Input: part model. Units: mm. Frame: model coordinates. A direction names the side the tool comes from. Give positions to 0.01 mm unless a question says otherwise; leave off trailing zeros. Write each loop counter-clockwise with the first axis right and the second up, starting at its lowest first coordinate (ties: lowest second). Pieces come first, ordered by that corner, then holes.
```python
from build123d import *

# Parameters (mm, degrees)
SKETCH1_W           = 58.42
SKETCH1_H           = 33.02
BOSS_EXTRUDE1_DEPTH = 7.62
BOSS_EXTRUDE2_DEPTH = 3.81
CUT_EXTRUDE1_DEPTH  = 35.407391648


with BuildPart() as part:
    # Sketch1 → Boss-Extrude1 (new body)
    with BuildSketch(Plane(origin=(0, 0, 0), x_dir=(1, 0, 0), z_dir=(0, 1, 0))):
        Rectangle(SKETCH1_W, SKETCH1_H)
    extrude(amount=BOSS_EXTRUDE1_DEPTH)

    # Sketch2 → Boss-Extrude2 (add)
    with BuildSketch(Plane.XZ):
        Polygon((5.08, -2.932939367), (5.08, 2.932939367), (0, 5.865878735), (-5.08, 2.932939367), (-5.08, -2.932939367), (0, -5.865878735), align=None)
    extrude(amount=BOSS_EXTRUDE2_DEPTH)

    # Sketch3 → Cut-Extrude1 (cut, through all)
    with BuildSketch(Plane(origin=(0, 0, 0), x_dir=(-1, 0, 0), z_dir=(0, -1, 0))):
        Polygon((26.162, -13.462), (26.162, 13.462), (8.128, 0), align=None)
        Polygon((8.128, -13.462), (21.066651169, -13.462), (8.128, -3.803570254), align=None)
        Polygon((21.066651169, 13.462), (8.128, 3.803570254), (8.128, 13.462), align=None)
        Polygon((-21.066651169, -13.462), (-8.128, -3.803570254), (-8.128, -13.462), align=None)
        Polygon((-8.128, 13.462), (-21.066651169, 13.462), (-8.128, 3.803570254), align=None)
        Polygon((-8.128, 0), (-26.162, -13.462), (-26.162, 13.462), align=None)
    extrude(amount=-CUT_EXTRUDE1_DEPTH, mode=Mode.SUBTRACT)


solid = part.part
```
Item 1: Section C-C (z = -11.5). Return loops of the section in (x, y).
Item 2: Pin query (flat end, axial travel): pin 1 (1.1 mm diameter, centred on y = -3, z = 0, fed in from +X); pin 2 (1.9 mm diameter, centred on y = -1, z = 0, fed in from -X). Return the tip coordinate at first contact, or that it passes through.
Item 3: Section B-B (x = -12.5). Return loops of the section in (y, z).
Item 4: Set-up query: faces 4 (the flat face through (-5.08, -2, 0)), 5 (the flat face through (2.576, -1.878, 4.379)), 6 (the flat face through (8.128, 4, -9)). Return all of +Z, -Z, +X, -X, +Y, -Y with unobstructed straight access to the full face (end or side cutting, diameter ignored); none if empty.
Item 5: Ray query, line 1 (Z direction, x = 16.5, y = 1.25); line 2 (Z direction, x = -14, y = 5); line 3 (X direction, y = 0.25, z = 3). Return the intervals inside material, ascending.
Item 6: Mould query, pull axis Z, two halves, no side actions, for faces 1 (the flat face through (14.69, 3.76, 8.7)), 2 (the flat face through (-7, 0, 0)), 3 (the flat face through (-2.576, -1.878, -4.379)). Classes: +Z half, -Z half, draft (parallel to the pull), parting line (faces both ways), or undercut.
Item 7: Section A-A (y = 6). Return loops of the section in (x, z), and give its area (3 significant figures).
Item 8: Section D-D (y = -2.5). Return loops of the section in (x, z).
Solved:
1. outline: (-29.21, 0) - (-26.16, 0) - (-26.16, 7.62) - (-29.21, 7.62) - close; (-23.53, 0) - (-18.44, 0) - (-18.44, 7.62) - (-23.53, 7.62) - close; (-8.13, 0) - (8.13, 0) - (8.13, 7.62) - (-8.13, 7.62) - close; (18.44, 0) - (23.53, 0) - (23.53, 7.62) - (18.44, 7.62) - close; (26.16, 0) - (29.21, 0) - (29.21, 7.62) - (26.16, 7.62) - close
2. pin 1: stops at x = 5.08
2. pin 2: stops at x = -5.08
3. outline: (0, -16.51) - (7.62, -16.51) - (7.62, -13.46) - (0, -13.46) - close; (0, -7.07) - (7.62, -7.07) - (7.62, -3.26) - (0, -3.26) - close; (0, 3.26) - (7.62, 3.26) - (7.62, 7.07) - (0, 7.07) - close; (0, 13.46) - (7.62, 13.46) - (7.62, 16.51) - (0, 16.51) - close
4. face 4: +Z, -Z, -X, -Y
4. face 5: +Z, +X, -Y
4. face 6: +Y, -Y
5. line 1: z = -16.51 to -13.46, -10.05 to -6.25, 6.25 to 10.05, 13.46 to 16.51
5. line 2: z = -16.51 to -13.46, -8.19 to -4.38, 4.38 to 8.19, 13.46 to 16.51
5. line 3: x = -29.21 to -26.16, -12.15 to 12.15, 26.16 to 29.21
6. face 1: undercut
6. face 2: draft
6. face 3: -Z half
7. outline: (-29.21, -16.51) - (29.21, -16.51) - (29.21, 16.51) - (-29.21, 16.51) - close; hole (-26.16, -13.46) - (-8.13, 0) - (-26.16, 13.46) - close; hole (-21.07, -13.46) - (-8.13, -13.46) - (-8.13, -3.8) - close; hole (-21.07, 13.46) - (-8.13, 3.8) - (-8.13, 13.46) - close; hole (8.13, -13.46) - (21.07, -13.46) - (8.13, -3.8) - close; hole (8.13, 0) - (26.16, -13.46) - (26.16, 13.46) - close; hole (8.13, 3.8) - (21.07, 13.46) - (8.13, 13.46) - close
7. area: 1,190 mm2
8. outline: (-5.08, -2.93) - (0, -5.87) - (5.08, -2.93) - (5.08, 2.93) - (0, 5.87) - (-5.08, 2.93) - close
